Source: three-view drawing plus pictorial views. Frame: mm from the lowest corner of the part. A direction names the side the tool comes from. Round coordinates to 2 decimals unless told otherwise and drop trailing zeros. Write each loop counter-clockwise with the first axis right and the second up, starting at its lowest first coordinate (ties: lowest second). Pieces come first, ordered by that corner, then holes. Notation, with made-up numbers: (-28, -16) -> (-2, -16) arc R20 cw to (-2, -3) -> close; hole circle Ø5 at (79, 49). An arc over 180 degrees is marked (long way). Put each result on its own line as item: value.
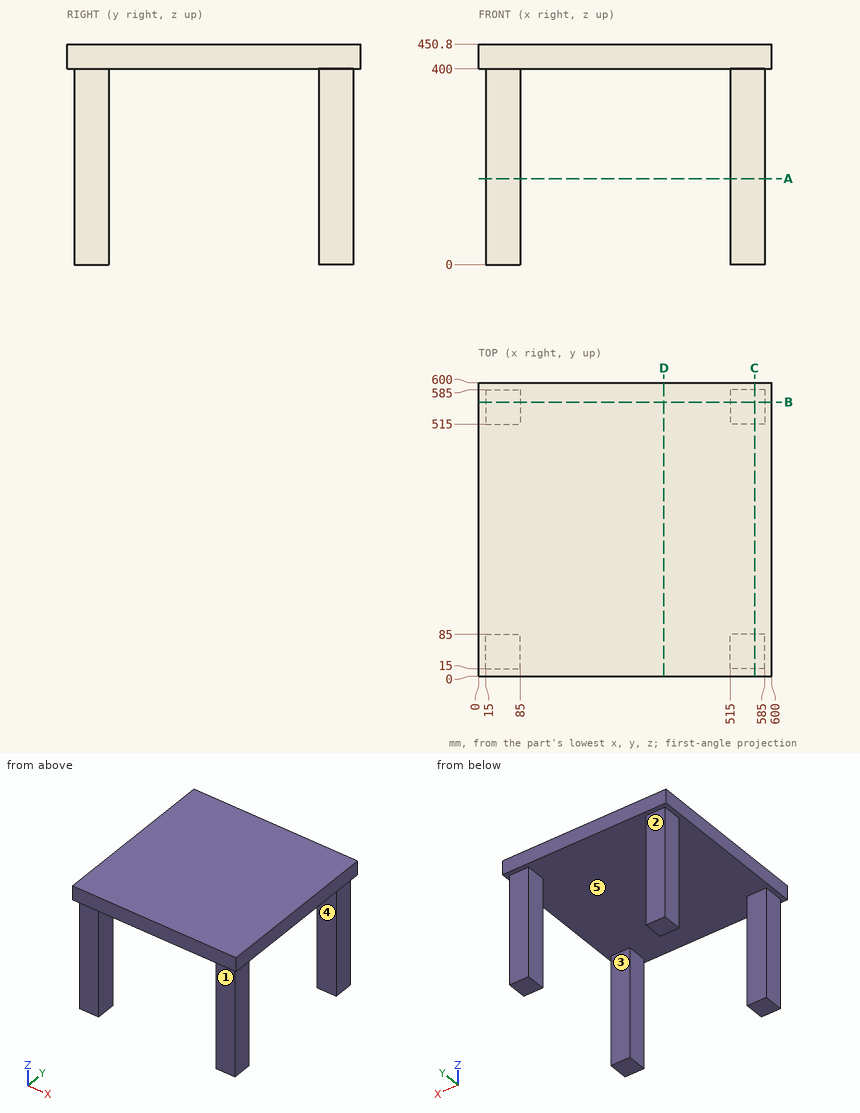
Q1. Cut plane A-A on z = 175.5. Output: boundary loops of the cut face in (x, y), and give its area (3 significant figures).
Ans:
outline: (15, 15) -> (85, 15) -> (85, 85) -> (15, 85) -> close; (15, 515) -> (85, 515) -> (85, 585) -> (15, 585) -> close; (515, 15) -> (585, 15) -> (585, 85) -> (515, 85) -> close; (515, 515) -> (585, 515) -> (585, 585) -> (515, 585) -> close
area: 19,600 mm^2
Q2. Cut plane D-D on x = 379. Output: boundary loops of the cut face in (y, z), and give its area (3 significant figures).
Ans:
outline: (0, 400) -> (600, 400) -> (600, 450.8) -> (0, 450.8) -> close
area: 30,500 mm^2
Q3. Draft query along X for the marked faces 4 and 5. Return one class per face: +X half, -X half, draft (parallel to the pull), parting line (faces both ways), or undercut.
Ans:
face 4: draft
face 5: undercut
Q4. Pin query (flat end, axial travel): pin 1 (21 mm diameter, centred on y = 562.5, z = 141, fed in from -X); pin 2 (21 mm diameter, centred on x = 44, z = 212.5, fed in from +Y); pin 3 (21 mm diameter, centred on y = 553.5, z = 216.5, fed in from +X). Return the tip coordinate at first contact, or that it passes through.
Ans:
pin 1: stops at x = 15
pin 2: stops at y = 585
pin 3: stops at x = 585
Q5. Material intervals for line 1 (X direction, y = 575.5, z = 95); line 2 (Z direction, x = 39.5, y = 305), sorted ascending. Write a range as [from, to].
Ans:
line 1: x = [15, 85], [515, 585]
line 2: z = [400, 450.8]
Q6. Cut plane B-B on y = 560. Output: boundary loops of the cut face in (x, z), and give its area (3 significant figures).
Ans:
outline: (0, 400) -> (15, 400) -> (15, 0) -> (85, 0) -> (85, 400) -> (515, 400) -> (515, 0) -> (585, 0) -> (585, 400) -> (600, 400) -> (600, 450.8) -> (0, 450.8) -> close
area: 86,500 mm^2
Q7. Reachability of the marked faces 1, 2 and 3 from +Z, -Z, +X, -X, +Y, -Y: full face, straight path, thin tool, end or side. Return the list, or none.
Ans:
face 1: -Z, +X, -X, -Y
face 2: -Z, +X, -X, +Y
face 3: -Z, +X, -X
